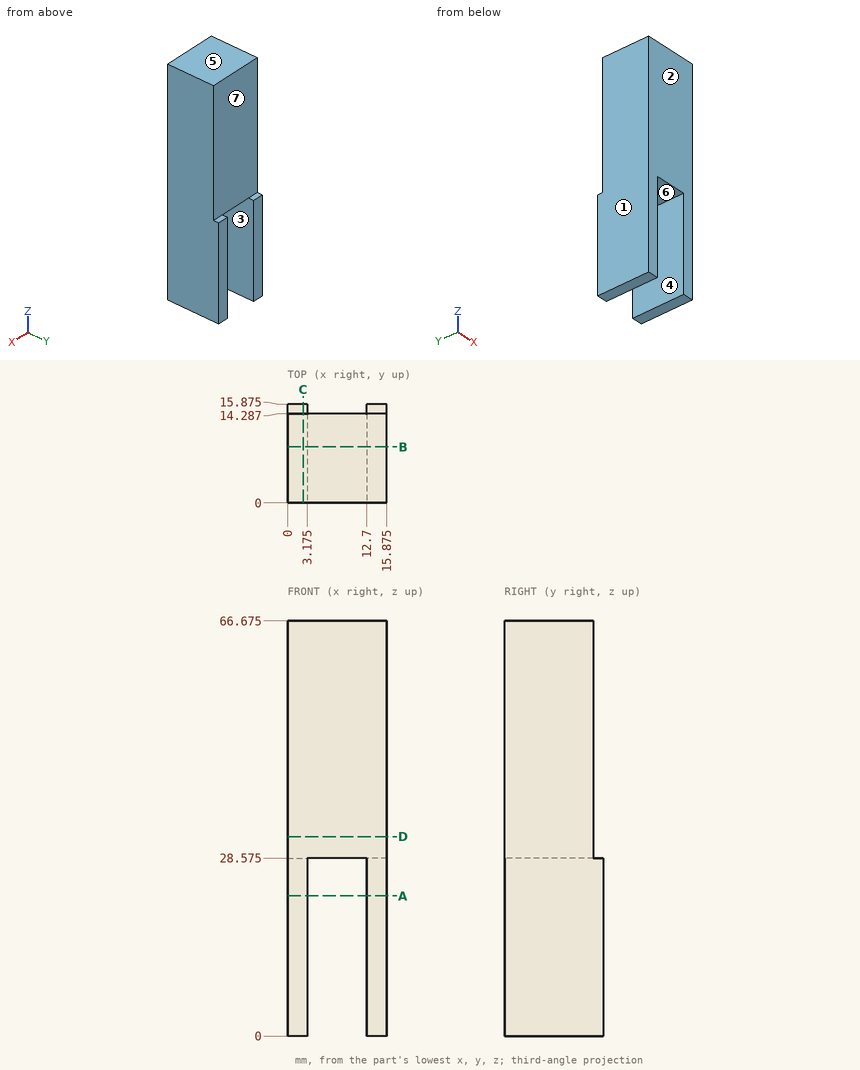
Could you check a few things on this drawing? It's one solid part, dimensions in mm from its lowest x, y, z. A direction names the side the tool comes from. Give positions to 0.01 mm unless a question says otherwise; leave off trailing zeros. Write each loop counter-clockwise with the first axis right and the second up, starting at its lowest first coordinate (ties: lowest second). Pieces come first, ordered by that corner, then holes. Notation, with made-up numbers: (24.5, -2.5) - (69.5, -2.5) arc R30 cw to (69.5, 34.5) - close; hole circle Ø11 at (42.5, 10). An arc over 180 degrees is marked (long way). Use CSV: the item, a comma, the result in double quotes. Start each with the question number.
Item 1: I want a section at C-C, the plane x = 2.5. Please give me the cut outline in (y, z) (1 decimal), then the cut area to 3 significant figures.
Item 2: For the marked faces 5, 6 and 7, which set-ups out of +Z, -Z, +X, -X, +Y, -Y let a thin tool reach every point of the face, with its end or its side?
Item 3: I want a section at D-D, the plane z = 32. Please give me the cut outline in (x, y) (1 decimal), then the cut area to 3 significant figures.
Item 4: I want a section at B-B, the plane y = 9. Please give me the cut outline in (x, z) (1 decimal).
Item 5: I'm going to push flat-ended pins straight in: pin 1 (3 mm diameter, centred on x = 2.5, z = 59, fed in from +Y); pin 2 (0.5 mm diameter, centred on x = 14, y = 15, fed in from +Z) (1 decimal); pin 3 (5 mm diameter, centred on x = 7.5, y = 4.5, fed in from -Z) (1 decimal). Where does each tip first touch, or does it pass through?
Item 6: If I drill on line 1 along X through (y, z) = (3.5, 12) (1 decimal); line 2 along Z through (x, y) = (11.5, 10.75) (1 decimal); line 3 along Y through (x, z) = (14.5, 46.5), over which ranges is the centre line in solid material (lowest first)?
Item 7: I want a section at A-A, the plane z = 22.5. Please give me the cut outline in (x, y) (1 decimal), then the cut area to 3 significant figures.
Item 8: If we mould it in two halves opening along X, with no side actions, what happens to the marked faces 1, 2, 3 and 4? For each: pulls with the +X half, pulls with the -X half, needs draft (parallel to the pull), parting line crosses it, or undercut.
Findings:
1,outline,"(0, 0) - (15.9, 0) - (15.9, 28.6) - (14.3, 28.6) - (14.3, 66.7) - (0, 66.7) - close"
1,area,"998 mm2"
2,face 5,"+Z, +X, -X, +Y, -Y"
2,face 6,"-Z, +Y, -Y"
2,face 7,"+Z, +X, -X, +Y"
3,outline,"(0, 0) - (15.9, 0) - (15.9, 14.3) - (0, 14.3) - close"
3,area,"227 mm2"
4,outline,"(0, 0) - (3.2, 0) - (3.2, 28.6) - (12.7, 28.6) - (12.7, 0) - (15.9, 0) - (15.9, 66.7) - (0, 66.7) - close"
5,pin 1,"stops at y = 14.29"
5,pin 2,"stops at z = 28.6"
5,pin 3,"stops at z = 28.6"
6,line 1,"x = 0 to 3.2, 12.7 to 15.9"
6,line 2,"z = 28.6 to 66.7"
6,line 3,"y = 0 to 14.29"
7,outline,"(0, 0) - (3.2, 0) - (3.2, 15.9) - (0, 15.9) - close; (12.7, 0) - (15.9, 0) - (15.9, 15.9) - (12.7, 15.9) - close"
7,area,"101 mm2"
8,face 1,"pulls with the -X half"
8,face 2,"needs draft"
8,face 3,"undercut"
8,face 4,"undercut"
